```python
from build123d import *


with BuildPart() as part:
    # Sweep1: sweep along a path in Sketch2
    with BuildLine(Plane(origin=(0, 0, 0), x_dir=(0, 0, -1), z_dir=(1, 0, 0))) as sweep1_path:
        Line((0, 0), (10, 0))
        Line((10, 0), (29.871437114, 2.264064275))
    # Sketch1 → Sweep1 (sweep)
    with BuildSketch(Plane.XY):
        Polygon((7.95, 0), (7.95, -2.04), (4.048, -6.152414984), (-4.048, -6.152414984), (-7.95, -2.04), (-7.95, 0), align=None)
    sweep(path=sweep1_path.line, transition=Transition.RIGHT)


solid = part.part
```
Could you check a few things on this model? Use its own coordinates, in mm. A direction names the side the tool comes from. Coordinates: 2 decimals unless noted, no trailing zeros. Write each loop counter-clockwise with the first axis right and the second up, starting at its lowest first coordinate (ties: lowest second). Pieces come first, ordered by that corner, then holes. Notation, with made-up numbers: (-30.5, 21) -> (-14.5, 21) arc R13 ccw to (-14.5, 45) -> close; hole circle Ø2 at (-13.75, -29.5). An arc over 180 degrees is marked (long way). Write item = value, one per line. Start each with the question number.
(1) Will these pins go through, and if not, where does the flat tip stop? pin 1 (5 mm diameter, centred on x = -2.5, z = -22.5, fed in from -Y); pin 2 (2 mm diameter, centred on x = 2.5, z = -26, fed in from -Y); pin 3 (1 mm diameter, centred on y = -5, z = -7, fed in from -X).
(2) I want a section at B-B (z = -6). Please give me the cut outline in (x, y).
(3) I want a section at C-C (y = 1.25). Please give me the cut outline in (x, z), plus the area to 3 significant figures.
(4) I need wall thicknesses on line 1 (Y direction, x = -2.75, z = -6); line 2 (Z direction, x = 2.75, y = -2.5); line 3 (Y direction, x = -6.5, z = -19.5). Which ranges of each line are inside material? Lowest first, please. Write a range as [from, to].
(5) Which directions (+Z, -Z, +X, -X, +Y, -Y) give clear straight access to the entire face, cutting with the end or side of a thin tool? Please do faces 1 (the face through (0, 0, -5)), 2 (the face through (5.972, -4.125, -5.247)).
(6) I want a section at A-A (x = 3.5). Please give me the cut outline in (y, z).
Result set:
q1.pin_1 = -5.05
q1.pin_2 = -4.48
q1.pin_3 = -5.62
q2.outline = (-7.95, -2.04) -> (-4.05, -6.15) -> (4.05, -6.15) -> (7.95, -2.04) -> (7.95, 0) -> (-7.95, 0) -> close
q3.outline = (-7.95, -29.99) -> (7.95, -29.99) -> (7.95, -20.97) -> (-7.95, -20.97) -> close
q3.area = 143 mm2
q4.line_1 = [-6.15, 0]
q4.line_2 = [-30.41, 0]
q4.line_3 = [-2.51, 1.08]
q5.face_1 = +Z, +X, -X, +Y
q5.face_2 = +Z, -Z, +X, -Y
q6.outline = (-6.15, -10.35) -> (-3.85, -30.57) -> (2.26, -29.87) -> (0, -10) -> (0, 0) -> (-6.15, 0) -> close
